Work out the finished part from the listing and answer in its coordinate system (mm). Face numbers are marked on the shaded views. A direction names the side the tool comes from. Give positions to 0.01 mm unless a question says otherwise; leave off trailing zeros. Write each loop counter-clockwise with the first axis right and the second up, starting at its lowest first coordinate (ties: lowest second). Pieces come first, ordered by that corner, then holes.
1) Find section D-D (x = 2). Determine the outline of the cut face in (y, z).
2) Find section A-A (z = 3.5). Determine the outline of the cut face in (x, y).
3) Given pin 1 Ø0.5 at (x, y) = (0, -0.5) entering from +Z; pin 2 Ø0.6 at (y, z) = (-1, -1) entering from +X; pin 3 Ø0.6 at (y, z) = (-1.5, -1) entering from -X, each flat-ended and moving along its own axis, determine where each tip first touches the part or whether it passes through.
4) Find section C-C (y = -1.25). Determine the outline of the cut face in (x, z), plus the area to 3 significant figures.
5) Straight lines are drawn through the part: probe 1 along X at (y, z) = (-0.15, 2.5); probe 2 along Z at (x, y) = (-2, 1.35); probe 3 along Z at (x, y) = (0, -0.7). For each, find the intervals that lie inside material, in ascending order.
6) Determine the mould class of the marked faces 1, 2 and 3 for opening direction X: pulls with the +X half, pulls with the -X half, needs draft (parallel to the pull), parting line crosses it, or undercut.
7) Find section B-B (z = -0.5). Determine the outline of the cut face in (x, y).
8) A tool of negligible diameter and unlimited length cuts with its end or side. For the marked faces 4, 5 and 6, from which of +Z, -Z, +X, -X, +Y, -Y can it reach the whole face along a straight path? Write none if from no direction.
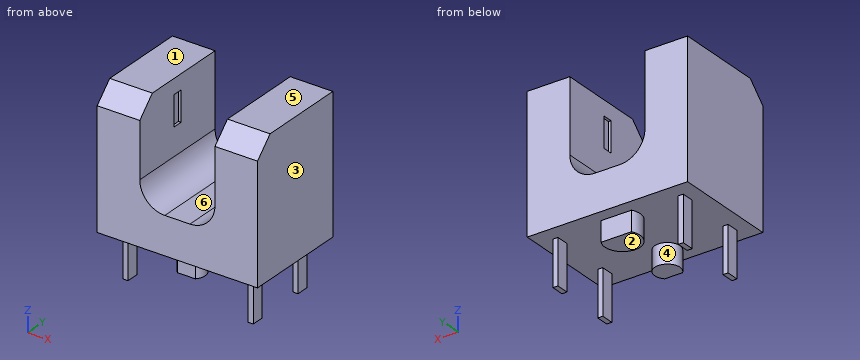
```python
from build123d import *

# Parameters (mm, degrees)
F0_W      = 6.4
F0_H      = 4.2
F1_DEPTH  = 5.4
F3_DEPTH  = 4.2
F4_SIZE   = 0.7
F5_W      = 0.4
F5_H      = 1.2
F6_DEPTH  = 1.6
F8_DEPTH  = 0.8
F9_W      = 0.2
F9_H      = 0.5
F10_DEPTH = 1.8


with BuildPart() as f1:
    # F0 (on Top) → F1 (new body)
    with BuildSketch(Plane.XY):
        Rectangle(F0_W, F0_H)
    extrude(amount=F1_DEPTH)

    # F2 (on face) → F3 (cut, through all)
    with BuildSketch(Plane.XZ.offset(2.1)):
        with BuildLine():
            Line((1.5, 2.5), (1.5, 5.4))
            Line((1.5, 5.4), (-1.5, 5.4))
            Line((-1.5, 5.4), (-1.5, 2.5))
            ThreePointArc((-1.5, 2.5), (-1.207107, 1.792893), (-0.5, 1.5))
            Line((-0.5, 1.5), (0.5, 1.5))
            ThreePointArc((0.5, 1.5), (1.207107, 1.792893), (1.5, 2.5))
        make_face()
    extrude(amount=-F3_DEPTH, mode=Mode.SUBTRACT)

    # F4
    f4_edges = [f1.edges().sort_by_distance(p)[0] for p in [
        (2.35, -2.1, 5.4),
        (-2.35, -2.1, 5.4),
    ]]
    chamfer(f4_edges, length=F4_SIZE)

    # F5 (on Right) → F6 (cut, symmetric)
    with BuildSketch(Plane.YZ):
        with Locations((0, 4.2)):
            Rectangle(F5_W, F5_H)
    extrude(amount=F6_DEPTH, both=True, mode=Mode.SUBTRACT)

    # F7 (on face) → F8 (join)
    with BuildSketch(Plane(origin=(0, 0, 0), x_dir=(1, 0, 0), z_dir=(0, 0, -1))):
        with BuildLine():
            Line((0.357071, 1.6), (-0.357071, 1.6))
            ThreePointArc((-0.357071, 1.6), (0, 0.75), (0.357071, 1.6))
        make_face()
        with BuildLine():
            Line((-0.606218, -1.6), (0.606218, -1.6))
            ThreePointArc((0.606218, -1.6), (0, -0.55), (-0.606218, -1.6))
        make_face()
    extrude(amount=F8_DEPTH)

    # F9 (on face) → F10 (join)
    with BuildSketch(Plane(origin=(0, 0, 0), x_dir=(1, 0, 0), z_dir=(0, 0, -1))):
        with Locations((-2.5, 1.25)):
            Rectangle(F9_W, F9_H)
        with Locations((-2.5, -1.25)):
            Rectangle(F9_W, F9_H)
        with Locations((2.5, 1.25)):
            Rectangle(F9_W, F9_H)
        with Locations((2.5, -1.25)):
            Rectangle(F9_W, F9_H)
    extrude(amount=F10_DEPTH)


solid = f1.part
```
Results:
1. outline: (-2.1, 0) - (2.1, 0) - (2.1, 5.4) - (-1.4, 5.4) - (-2.1, 4.7) - close
2. outline: (-3.2, -2.1) - (-1.5, -2.1) - (-1.5, 2.1) - (-3.2, 2.1) - close; (1.5, -2.1) - (3.2, -2.1) - (3.2, 2.1) - (1.5, 2.1) - close
3. pin 1: stops at z = 1.5
3. pin 2: stops at x = 2.6
3. pin 3: stops at x = -2.6
4. outline: (-3.2, 0) - (-2.6, 0) - (-2.6, -1.8) - (-2.4, -1.8) - (-2.4, 0) - (-0.5, 0) - (-0.5, -0.8) - (0.5, -0.8) - (0.5, 0) - (2.4, 0) - (2.4, -1.8) - (2.6, -1.8) - (2.6, 0) - (3.2, 0) - (3.2, 5.4) - (1.5, 5.4) - (1.5, 2.5) arc R1 cw to (0.5, 1.5) - (-0.5, 1.5) arc R1 cw to (-1.5, 2.5) - (-1.5, 5.4) - (-3.2, 5.4) - close
4. area: 24.8 mm2
5. probe 1: x = -3.2 to -1.5, 1.5 to 3.2
5. probe 2: z = 0 to 5.4
5. probe 3: z = 0 to 1.5
6. face 1: needs draft
6. face 2: undercut
6. face 3: pulls with the +X half
7. outline: (-2.6, -1.5) - (-2.4, -1.5) - (-2.4, -1) - (-2.6, -1) - close; (-2.6, 1) - (-2.4, 1) - (-2.4, 1.5) - (-2.6, 1.5) - close; (-0.61, 1.6) arc R0.7 ccw (long way) to (0.61, 1.6) - close; (-0.36, -1.6) - (0.36, -1.6) arc R0.5 ccw (long way) to start; (2.4, -1.5) - (2.6, -1.5) - (2.6, -1) - (2.4, -1) - close; (2.4, 1) - (2.6, 1) - (2.6, 1.5) - (2.4, 1.5) - close
8. face 4: -Z
8. face 5: +Z, +X, -X, +Y, -Y
8. face 6: +Z, +Y, -Y
